Autodesk Inventor part; units mm, degrees
ref_plane "YZ Plane" through (0, 0, 0) normal (1, 0, 0) x (0, 1, 0)
ref_plane "XZ Plane" through (0, 0, 0) normal (0, 1, 0) x (-1, 0, 0)
ref_plane "XY Plane" through (0, 0, 0) normal (0, 0, 1) x (1, 0, 0)
sketch "Sketch1" plane through (0, 0, 0) normal (0, 1, 0) x (-1, 0, 0)
  line L0 (11, -8.5) -> (-11, -8.5)
  line L1 (-11, -8.5) -> (-11, 8.5)
  line L2 (-11, 8.5) -> (11, 8.5)
  line L3 (11, 8.5) -> (11, -8.5)
  line L4 (11, -8.5) -> (-11, 8.5) construction
  line L5 (-11, -8.5) -> (11, 8.5) construction
  point P0 (0, 0)
  dimension "d0" = 22
  dimension "d1" = 17
extrude "Extrusion1" add sketch "Sketch1" along normal blind 5
sketch "Sketch2" plane through (0, 5, 0) normal (0, 1, 0) x (1, 0, 0)
  circle A0 centre (0, 0) radius 6
  circle A1 centre (0, 0) radius 3.05
  dimension "d4" = 12
  dimension "d5" = 6.1
extrude "Extrusion2" add sketch "Sketch2" along normal blind 10
properties part number "imusupport"
Part model, mm, in its own coordinate system. A direction names the side the tool comes from. Give positions to 0.01 mm unless a question says otherwise; leave off trailing zeros. Write each loop counter-clockwise with the first axis right and the second up, starting at its lowest first coordinate (ties: lowest second). Pieces come first, ordered by that corner, then holes. Notation, with made-up numbers: M 9.25,6.5 L 56.25,6.5 A32 cw 56.25,44.5 Z; hole C 85,-32 d11. An arc over 180 degrees is marked long. Use CSV: the item, a comma, the result in double quotes.
Item 1: Slice it at C-C on y = 6.75. Write the cut outline in (x, z).
Taken from the geometry:
outline,"C 0,0 d12; hole C 0,0 d6.1"
Item 2: Which spindle directions (+Z, -Z, +X, -X, +Y, -Y) get a long thin tool onto all of the face, cutting with end or side? Do faces 1 (the face through (0, 2, -8.5)), 2 (the face through (-3.047, 9.93, 0.134)). Say none if no direction does.
Taken from the geometry:
face 1,"-Z, +X, -X, +Y, -Y"
face 2,"+Y"
Item 3: Slice it at B-B on x = 0. Write the cut outline in (y, z), plus the area to 3 significant figures.
Taken from the geometry:
outline,"M 0,-8.5 L 5,-8.5 L 5,-6 L 15,-6 L 15,-3.05 L 5,-3.05 L 5,3.05 L 15,3.05 L 15,6 L 5,6 L 5,8.5 L 0,8.5 Z"
area,"144 mm²"
Item 4: Slice it at A-A on z = 0. Write the cut outline in (x, y).
Taken from the geometry:
outline,"M -11,0 L 11,0 L 11,5 L 6,5 L 6,15 L 3.05,15 L 3.05,5 L -3.05,5 L -3.05,15 L -6,15 L -6,5 L -11,5 Z"
Item 5: Slice it at D-D on z = -4.5. Write the cut outline in (x, y).
Taken from the geometry:
outline,"M -11,0 L 11,0 L 11,5 L 3.97,5 L 3.97,15 L -3.97,15 L -3.97,5 L -11,5 Z"
Item 6: Drill centre lines: probe 1 along Z at (x, y) = (0, 11); probe 2 along Y at (x, z) = (5.75, -2.25). Where is each one in solid material? Low to high.
Taken from the geometry:
probe 1,"z = -6 to -3.05, 3.05 to 6"
probe 2,"y = 0 to 5"
Item 7: Pin check, flat tips, straight feed: P1, Ø5, axis at x = 0, z = 0, coming from the +Y side; P2, Ø4, axis at x = -6.5, y = 11, coming from the +Z side; P3, Ø4, axis at x = 2, y = 13, coming from the -Z side. Stop position of each tip, or through.
Taken from the geometry:
P1,"stops at y = 5"
P2,"stops at z = 3.97"
P3,"stops at z = -6"
